```python
from build123d import *
from build123d.topology import SkipClean

# Parameters (mm, degrees)
SKETCH1_R           = 110.731806219
SKETCH1_R_2         = 107.731806219
BOSS_EXTRUDE1_DEPTH = 2
BOSS_EXTRUDE3_DEPTH = 30


with BuildPart() as part:
    # Sketch1 → Boss-Extrude1 (new body)
    with BuildSketch(Plane.XY):
        Circle(SKETCH1_R)
        Circle(SKETCH1_R_2, mode=Mode.SUBTRACT)
    extrude(amount=BOSS_EXTRUDE1_DEPTH)

    # Sketch3 → Boss-Extrude3 (add)
    with SkipClean():  # the faces are left unmerged after this step: merging them gives an invalid solid
        with BuildSketch(Plane.XY):
            with BuildLine():
                Line((1, 107.727164964), (1, 110.727290712))
                ThreePointArc((1, 110.727290712), (0, 110.731806219), (-1, 110.727290712))
                Line((-1, 110.727290712), (-1, 107.727164964))
                ThreePointArc((-1, 107.727164964), (0, 107.731806219), (1, 107.727164964))
            make_face()
            with BuildLine():
                Line((107.727164964, 1), (110.727290712, 1))
                ThreePointArc((110.727290712, 1), (110.731806219, 0), (110.727290712, -1))
                Line((110.727290712, -1), (107.727164964, -1))
                ThreePointArc((107.727164964, -1), (107.731806219, 0), (107.727164964, 1))
            make_face()
            with BuildLine():
                Line((76.881715645, -75.467502083), (79.003124906, -77.588911344))
                ThreePointArc((79.003124906, -77.588911344), (78.29921107, -78.29921107), (77.588911344, -79.003124906))
                Line((77.588911344, -79.003124906), (75.467502083, -76.881715645))
                ThreePointArc((75.467502083, -76.881715645), (76.177890727, -76.177890727), (76.881715645, -75.467502083))
            make_face()
            with BuildLine():
                Line((1, -107.727164964), (1, -110.727290712))
                ThreePointArc((1, -110.727290712), (0, -110.731806219), (-1, -110.727290712))
                Line((-1, -110.727290712), (-1, -107.727164964))
                ThreePointArc((-1, -107.727164964), (0, -107.731806219), (1, -107.727164964))
            make_face()
            with BuildLine():
                Line((-75.467502083, -76.881715645), (-77.588911344, -79.003124906))
                ThreePointArc((-77.588911344, -79.003124906), (-78.29921107, -78.29921107), (-79.003124906, -77.588911344))
                Line((-79.003124906, -77.588911344), (-76.881715645, -75.467502083))
                ThreePointArc((-76.881715645, -75.467502083), (-76.177890727, -76.177890727), (-75.467502083, -76.881715645))
            make_face()
            with BuildLine():
                Line((-107.727164964, -1), (-110.727290712, -1))
                ThreePointArc((-110.727290712, -1), (-110.731806219, 0), (-110.727290712, 1))
                Line((-110.727290712, 1), (-107.727164964, 1))
                ThreePointArc((-107.727164964, 1), (-107.731806219, 0), (-107.727164964, -1))
            make_face()
            with BuildLine():
                Line((-76.881715645, 75.467502083), (-79.003124906, 77.588911344))
                ThreePointArc((-79.003124906, 77.588911344), (-78.29921107, 78.29921107), (-77.588911344, 79.003124906))
                Line((-77.588911344, 79.003124906), (-75.467502083, 76.881715645))
                ThreePointArc((-75.467502083, 76.881715645), (-76.177890727, 76.177890727), (-76.881715645, 75.467502083))
            make_face()
            with BuildLine():
                Line((99.144239373, 42.14928078), (101.915994147, 43.297379199))
                ThreePointArc((101.915994147, 43.297379199), (102.302849363, 42.375227676), (102.681361012, 41.449620134))
                Line((102.681361012, 41.449620134), (99.909606238, 40.301521715))
                ThreePointArc((99.909606238, 40.301521715), (99.531210766, 41.227177379), (99.144239373, 42.14928078))
            make_face()
            with BuildLine():
                Line((40.301521715, 99.909606238), (41.449620134, 102.681361012))
                ThreePointArc((41.449620134, 102.681361012), (42.375227676, 102.302849363), (43.297379199, 101.915994147))
                Line((43.297379199, 101.915994147), (42.14928078, 99.144239373))
                ThreePointArc((42.14928078, 99.144239373), (41.227177379, 99.531210766), (40.301521715, 99.909606238))
            make_face()
        extrude(amount=BOSS_EXTRUDE3_DEPTH)


solid = part.part
```
Geometry: final body of the model. Coordinates: model frame, mm. Give positions to 0.01 mm unless a question says otherwise; leave off trailing zeros. Order: outer loops, then holes, each group sorted by start corner. A loop starts at its lowest first (then second) coordinate and runs counter-clockwise, first axis right, second up. Notation, with made-up numbers: (89.5, 18) -> (113.5, 18) arc R15 cw to (113.5, 27) -> close; hole circle Ø8 at (-3, 16.5). An arc over 180 degrees is marked (long way). Write each question's results on one line, items separated by ' | '. Start each with the question number.
1) Line query: line 1 (Y direction, x = 0, z = 1.4); line 2 (X direction, y = 41, z = 7.5) (3 decimals). Output: solid intervals per line, ascending. Write a range as from..to.
2) First-contact query: pin 1 (1.5 mm diameter, centred on x = -108.5, z = 16, fed in from -Y); pin 2 (5 mm diameter, centred on y = 76, z = 15, fed in from +X); pin 3 (8.5 mm diameter, centred on x = 105.5, y = 18.5, fed in from +Z); pin 4 (3 mm diameter, centred on x = 19, y = 103, fed in from +Z). Flat tips, straight axial feed; report the tip coordinate or a pass-through.
3) Section C-C (z = 6.25). Count the separate pieces of the cut face and the enclosed holes in it, then the cut area to 3 significant figures.
4) Section B-B (x = -4). Return loops of the section in (y, z), then the cut area to 3 significant figures.
5) Section A-A (y = 95). Return loops of the section in (x, z), then the cut area to 3 significant figures.
Calculated:
1) line 1: -110.73..-107.73, 107.73..110.73 | line 2: 99.625..101.596
2) pin 1: y = -1 | pin 2: x = -75.47 | pin 3: z = 2 | pin 4: through
3) separate pieces: 9 | enclosed holes: 0 | area: 54.0 mm2
4) outline: (-110.66, 0) -> (-107.66, 0) -> (-107.66, 2) -> (-110.66, 2) -> close; (107.66, 0) -> (110.66, 0) -> (110.66, 2) -> (107.66, 2) -> close | area: 12.0 mm2
5) outline: (-56.89, 0) -> (-50.8, 0) -> (-50.8, 2) -> (-56.89, 2) -> close; (50.8, 0) -> (56.89, 0) -> (56.89, 2) -> (50.8, 2) -> close | area: 24.3 mm2
